Check sheet for the modelled part. Datum: model origin and axes. Units: mm. A direction names the side the tool comes from. Coordinates: 2 decimals unless noted, no trailing zeros. Write each loop counter-clockwise with the first axis right and the second up, starting at its lowest first coordinate (ties: lowest second). Pieces come first, ordered by that corner, then holes. Notation, with made-up numbers: (69.25, 80) -> (73.25, 80) arc R21 cw to (73.25, 95) -> close; hole circle Ø7 at (-18, 72). An arc over 180 degrees is marked (long way). One line per item, written item: value. Start each with the question number.
1) Sectioned sample at B-B on y = 0. Enter the section's corners in (x, z).
2) Sectioned sample at C-C on x = 0. Enter the section's corners in (y, z).
3) Set-up check for faces 1 (the flat face through (-49, 26, 0)), 2 (the flat face through (-2.5, 16, 28)), 3 (the flat face through (14, -6, 53)), 4 (the cylindrical face through (1.32, -29.97, 32.72)), 5 (the flat face through (-11, -11, 3)): record each of +Z, -Z, +X, -X, +Y, -Y from which the full face is reachable in a straight line by a thin tool's end or side.
4) Sectioned sample at A-A on z = 19.5. Enter the section's corners in (x, y).
5) Draft check along X on faces 6 (the flat face through (-49, -26, 23)), 7 (the cylindrical face through (2.64, -59.94, 11.34)), 8 (the flat face through (2.5, 16, 28)). Enter one of: +X half, -X half, draft (parallel to the pull), parting line (faces both ways), or undercut.
6) Sectioned sample at D-D on y = 40. Enter the section's corners in (x, z).
7) Gauge pin test, flat ends, axial feed: P1, Ø2, axis at x = 26.5, z = 21, coming from the -Y side; P2, Ø1.5, axis at y = 4, z = 35.5, coming from the -X side; P3, Ø4, axis at x = 24, y = 28, coming from the +Z side. Record the tip position at first contact, or that the pin passes through.
8) Scan lines: line 1 along X through (y, z) = (0, 16.5); line 2 along X through (y, z) = (0, 2.2); line 3 along X through (y, z) = (0, 9.75). Record each from-to range of solid material in increasing order. Write a range as [from, to].
```python
from build123d import *

# Parameters (mm, degrees)
SKETCH2_W            = 5
SKETCH2_H            = 5
CUT_EXTRUDE1_DEPTH   = 54
M8_CLEARANCE_HOLE2_D = 9
CIRPATTERN1_COUNT    = 4


with BuildPart() as part:
    # Sketch1 → Revolve1 (revolve)
    with BuildSketch(Plane(origin=(0, 0, 0), x_dir=(0, 0, -1), z_dir=(1, 0, 0))):
        Polygon((-3, 15), (-53, 15), (-53, 30), (-13, 30), (-13, 55), (-23, 55), (-23, 60), (0, 60), (0, 55), (-3, 55), (-3, 33.885514375), align=None)
    revolve(axis=Axis((0, 0, 0), (0, 0, -1)))

    # Sketch2 → Cut-Extrude1 (cut, through all)
    with BuildSketch(Plane.XY.offset(53)):
        with Locations((0, 15)):
            Rectangle(SKETCH2_W, SKETCH2_H)
    extrude(amount=-CUT_EXTRUDE1_DEPTH, mode=Mode.SUBTRACT)

    # M8 Clearance Hole2 (through all)
    with Locations(Plane.XY.offset(13)):
        with Locations((0, 40)):
            m8_clearance_hole2 = Hole(M8_CLEARANCE_HOLE2_D / 2)

    # CirPattern1: M8 Clearance Hole2 ×4 about axis
    cirpattern1_axis = Axis((0, 0, 0), (0, 0, 1))
    for i in range(1, CIRPATTERN1_COUNT):
        add(m8_clearance_hole2.rotate(cirpattern1_axis, i * 360 / CIRPATTERN1_COUNT), mode=Mode.SUBTRACT)


solid = part.part
```
Answers:
1. outline: (-60, 0) -> (-55, 0) -> (-55, 3) -> (-44.5, 3) -> (-44.5, 13) -> (-55, 13) -> (-55, 23) -> (-60, 23) -> close; (-35.5, 3) -> (-15, 3) -> (-15, 53) -> (-30, 53) -> (-30, 13) -> (-35.5, 13) -> close; (15, 3) -> (35.5, 3) -> (35.5, 13) -> (30, 13) -> (30, 53) -> (15, 53) -> close; (44.5, 3) -> (55, 3) -> (55, 0) -> (60, 0) -> (60, 23) -> (55, 23) -> (55, 13) -> (44.5, 13) -> close
2. outline: (-60, 0) -> (-55, 0) -> (-55, 3) -> (-44.5, 3) -> (-44.5, 13) -> (-55, 13) -> (-55, 23) -> (-60, 23) -> close; (-35.5, 3) -> (-15, 3) -> (-15, 53) -> (-30, 53) -> (-30, 13) -> (-35.5, 13) -> close; (17.5, 3) -> (35.5, 3) -> (35.5, 13) -> (30, 13) -> (30, 53) -> (17.5, 53) -> close; (44.5, 3) -> (55, 3) -> (55, 0) -> (60, 0) -> (60, 23) -> (55, 23) -> (55, 13) -> (44.5, 13) -> close
3. face 1: -Z, +X, -X, +Y, -Y
3. face 2: +Z, -Z
3. face 3: +Z, +X, -X, +Y, -Y
3. face 4: +Z
3. face 5: -Z
4. outline: circle Ø120 at (0, 0); circle Ø60 at (0, 0); hole circle Ø110 at (0, 0); hole (-2.5, 14.79) arc R15 ccw (long way) to (2.5, 14.79) -> (2.5, 17.5) -> (-2.5, 17.5) -> close
5. face 6: draft
5. face 7: parting line
5. face 8: undercut
6. outline: (-44.72, 0) -> (-37.75, 0) -> (-37.75, 3) -> (-4.5, 3) -> (-4.5, 13) -> (-37.75, 13) -> (-37.75, 23) -> (-44.72, 23) -> close; (4.5, 3) -> (37.75, 3) -> (37.75, 0) -> (44.72, 0) -> (44.72, 23) -> (37.75, 23) -> (37.75, 13) -> (4.5, 13) -> close
7. P1: stops at y = -54.31
7. P2: stops at x = -29.82
7. P3: stops at z = 13
8. line 1: x = [-60, -55], [-30, -15], [15, 30], [55, 60]
8. line 2: x = [-60, -55], [55, 60]
8. line 3: x = [-60, -44.5], [-35.5, -15], [15, 35.5], [44.5, 60]
